Geometry: final body of the model. Coordinates: model frame, mm. Face numbers are marked on the shaded views. A direction names the side the tool comes from. Give positions to 0.01 mm unless a question says otherwise; leave off trailing zeros. Write each loop counter-clockwise with the first axis right and the second up, starting at its lowest first coordinate (ties: lowest second). Pieces come first, ordered by that corner, then holes. Notation, with made-up numbers: (78.5, 59) -> (108.5, 59) arc R11 cw to (108.5, 78) -> close; hole circle Ø7 at (-40, -22). An arc over 180 degrees is marked (long way). Answer as a JSON object with one key per item and string values.
from build123d import *

# Parameters (mm, degrees)
SKETCH1_W           = 154
SKETCH1_H           = 116
BOSS_EXTRUDE1_DEPTH = 70
SKETCH2_W           = 150
SKETCH2_H           = 102
CUT_EXTRUDE1_DEPTH  = 68
SKETCH3_W           = 140
SKETCH3_H           = 5
CUT_EXTRUDE2_DEPTH  = 68
SKETCH5_W           = 70
SKETCH5_H           = 56
CUT_EXTRUDE4_DEPTH  = 5
SKETCH17_W          = 9
SKETCH17_H          = 11
CUT_EXTRUDE12_DEPTH = 178.110135227
FILLET1_R           = 2
FILLET3_R           = 5
FILLET4_R           = 3
FILLET5_R           = 3
FILLET6_R           = 3
FILLET7_R           = 3
FILLET9_R           = 3
FILLET11_R          = 2
FILLET12_R          = 3
FILLET13_R          = 2
SKETCH18_W          = 154
SKETCH18_H          = 116
CUT_EXTRUDE13_DEPTH = 4
SKETCH19_R          = 5
CUT_EXTRUDE14_DEPTH = 4
SKETCH20_R          = 3.5
BOSS_EXTRUDE3_DEPTH = 19.5
SKETCH22_R          = 3.5
BOSS_EXTRUDE4_DEPTH = 18
SKETCH24_R          = 3.25
CUT_EXTRUDE17_DEPTH = 149.882504009
SKETCH25_R          = 3.25
CUT_EXTRUDE18_DEPTH = 176.567650779
SKETCH6_R           = 1.5
CUT_EXTRUDE19_DEPTH = 60
SKETCH26_R          = 2.1
CUT_EXTRUDE20_DEPTH = 10
SKETCH23_R          = 1.5
CUT_EXTRUDE21_DEPTH = 15
SKETCH27_R          = 2.1
CUT_EXTRUDE22_DEPTH = 10
SKETCH21_R          = 1.5
CUT_EXTRUDE23_DEPTH = 15
SKETCH28_R          = 2.1
CUT_EXTRUDE24_DEPTH = 10


with BuildPart() as part:
    # Sketch1 → Boss-Extrude1 (new body)
    with BuildSketch(Plane(origin=(0, 0, 0), x_dir=(1, 0, 0), z_dir=(0, 1, 0))):
        Rectangle(SKETCH1_W, SKETCH1_H)
    extrude(amount=BOSS_EXTRUDE1_DEPTH)

    # Sketch2 → Cut-Extrude1 (cut)
    with BuildSketch(Plane(origin=(0, 70, 0), x_dir=(1, 0, 0), z_dir=(0, 1, 0))):
        Rectangle(SKETCH2_W, SKETCH2_H)
    extrude(amount=-CUT_EXTRUDE1_DEPTH, mode=Mode.SUBTRACT)

    # Sketch3 → Cut-Extrude2 (cut)
    with BuildSketch(Plane(origin=(0, 70, 0), x_dir=(1, 0, 0), z_dir=(0, 1, 0))):
        with Locations((0, 53.5)):
            Rectangle(SKETCH3_W, SKETCH3_H)
    extrude(amount=-CUT_EXTRUDE2_DEPTH, mode=Mode.SUBTRACT)

    # Sketch5 → Cut-Extrude4 (cut)
    with BuildSketch(Plane.XY.offset(58)):
        with Locations((35, 35)):
            Rectangle(SKETCH5_W, SKETCH5_H)
        with Locations((-35, 35)):
            Rectangle(SKETCH5_W, SKETCH5_H)
    extrude(amount=-CUT_EXTRUDE4_DEPTH, mode=Mode.SUBTRACT)

    # Sketch17 → Cut-Extrude12 (cut, through all)
    with BuildSketch(Plane.ZY.offset(-75)):
        with Locations((45.3, 27.5)):
            Rectangle(SKETCH17_W, SKETCH17_H)
    extrude(amount=-CUT_EXTRUDE12_DEPTH, mode=Mode.SUBTRACT)

    # Fillet1
    fillet1_edges = [part.edges().sort_by_distance(p)[0] for p in [
        (77, 27.5, 49.8),
        (77, 22, 45.3),
        (77, 27.5, 40.8),
        (77, 33, 45.3),
    ]]
    fillet(fillet1_edges, radius=FILLET1_R - 0.0001)  # a hair under: the kernel refuses the full size

    # Fillet3
    fillet3_edges = [part.edges().sort_by_distance(p)[0] for p in [
        (0, 7, 53),
        (70, 35, 53),
        (-70, 35, 53),
        (0, 63, 53),
    ]]
    fillet(fillet3_edges, radius=FILLET3_R - 0.0001)  # a hair under: the kernel refuses the full size

    # Fillet4
    fillet4_edges = [part.edges().sort_by_distance(p)[0] for p in [
        (77, 35, 58),
    ]]
    fillet(fillet4_edges, radius=FILLET4_R)

    # Fillet5
    fillet5_edges = [part.edges().sort_by_distance(p)[0] for p in [
        (-77, 35, 58),
    ]]
    fillet(fillet5_edges, radius=FILLET5_R)

    # Fillet6
    fillet6_edges = [part.edges().sort_by_distance(p)[0] for p in [
        (-77, 35, -58),
    ]]
    fillet(fillet6_edges, radius=FILLET6_R)

    # Fillet7
    fillet7_edges = [part.edges().sort_by_distance(p)[0] for p in [
        (77, 35, -58),
    ]]
    fillet(fillet7_edges, radius=FILLET7_R)

    # Fillet9
    fillet9_edges = [part.edges().sort_by_distance(p)[0] for p in [
        (-70, 36, -51),
    ]]
    fillet(fillet9_edges, radius=FILLET9_R)

    # Fillet11
    fillet11_edges = [part.edges().sort_by_distance(p)[0] for p in [
        (-70, 36, -56),
    ]]
    fillet(fillet11_edges, radius=FILLET11_R - 0.0001)  # a hair under: the kernel refuses the full size

    # Fillet12
    fillet12_edges = [part.edges().sort_by_distance(p)[0] for p in [
        (70, 36, -51),
    ]]
    fillet(fillet12_edges, radius=FILLET12_R)

    # Fillet13
    fillet13_edges = [part.edges().sort_by_distance(p)[0] for p in [
        (70, 36, -56),
    ]]
    fillet(fillet13_edges, radius=FILLET13_R - 0.0001)  # a hair under: the kernel refuses the full size

    # Sketch18 → Cut-Extrude13 (cut)
    with BuildSketch(Plane(origin=(0, 70, 0), x_dir=(1, 0, 0), z_dir=(0, 1, 0))):
        Rectangle(SKETCH18_W, SKETCH18_H)
    extrude(amount=-CUT_EXTRUDE13_DEPTH, mode=Mode.SUBTRACT)

    # Sketch19 → Cut-Extrude14 (cut)
    with BuildSketch(Plane(origin=(0, 0, 51), x_dir=(-1, 0, 0), z_dir=(0, 0, -1))):
        with Locations((-13.5, 34)):
            Circle(SKETCH19_R)
        with Locations((4.25, 34)):
            Circle(SKETCH19_R)
        with Locations((22, 34)):
            Circle(SKETCH19_R)
    extrude(amount=-CUT_EXTRUDE14_DEPTH, mode=Mode.SUBTRACT)

    # Sketch20 → Boss-Extrude3 (add)
    with BuildSketch(Plane(origin=(0, 2, 0), x_dir=(1, 0, 0), z_dir=(0, 1, 0))):
        with Locations(Location((-60, -36, 0), (0, 0, 270))):
            Circle(SKETCH20_R)
        with Locations(Location((8, -40, 0), (0, 0, 270))):
            Circle(SKETCH20_R)
        with Locations(Location((-59, 33, 0), (0, 0, 270))):
            Circle(SKETCH20_R)
        with Locations(Location((20, 34, 0), (0, 0, 270))):
            Circle(SKETCH20_R)
    extrude(amount=BOSS_EXTRUDE3_DEPTH)

    # Sketch22 → Boss-Extrude4 (add)
    with BuildSketch(Plane(origin=(0, 2, 0), x_dir=(1, 0, 0), z_dir=(0, 1, 0))):
        with Locations(Location((50, 29, 0), (0, 0, 270))):
            Circle(SKETCH22_R)
        with Locations(Location((35, 3, 0), (0, 0, 270))):
            Circle(SKETCH22_R)
        with Locations(Location((67, 3, 0), (0, 0, 270))):
            Circle(SKETCH22_R)
        with Locations(Location((54, -44, 0), (0, 0, 270))):
            Circle(SKETCH22_R)
    extrude(amount=BOSS_EXTRUDE4_DEPTH)

    # Sketch24 → Cut-Extrude17 (cut, through all)
    with BuildSketch(Plane(origin=(0, 0, 51), x_dir=(-1, 0, 0), z_dir=(0, 0, -1))):
        with Locations((-35, 24.5)):
            Circle(SKETCH24_R)
    extrude(amount=-CUT_EXTRUDE17_DEPTH, mode=Mode.SUBTRACT)

    # Sketch25 → Cut-Extrude18 (cut, through all)
    with BuildSketch(Plane(origin=(-75, 0, 0), x_dir=(0, 0, -1), z_dir=(1, 0, 0))):
        with Locations((-44, 24.5)):
            Circle(SKETCH25_R)
        with Locations((41.2, 24.5)):
            Circle(SKETCH25_R)
    extrude(amount=-CUT_EXTRUDE18_DEPTH, mode=Mode.SUBTRACT)

    # Sketch6 → Cut-Extrude19 (cut)
    with BuildSketch(Plane(origin=(0, 70, 0), x_dir=(1, 0, 0), z_dir=(0, 1, 0))):
        with Locations(Location((73.5, 54.5, 0), (0, 0, 270))):
            Circle(SKETCH6_R)
        with Locations(Location((-73.5, 54.5, 0), (0, 0, 270))):
            Circle(SKETCH6_R)
        with Locations(Location((73.5, -54.5, 0), (0, 0, 270))):
            Circle(SKETCH6_R)
        with Locations(Location((-73.5, -54.5, 0), (0, 0, 270))):
            Circle(SKETCH6_R)
    extrude(amount=-CUT_EXTRUDE19_DEPTH, mode=Mode.SUBTRACT)

    # Sketch26 → Cut-Extrude20 (cut)
    with BuildSketch(Plane(origin=(0, 66, 0), x_dir=(1, 0, 0), z_dir=(0, 1, 0))):
        with Locations(Location((73.5, -54.5, 0), (0, 0, 270))):
            Circle(SKETCH26_R)
        with Locations(Location((73.5, 54.5, 0), (0, 0, 270))):
            Circle(SKETCH26_R)
        with Locations(Location((-73.5, 54.5, 0), (0, 0, 270))):
            Circle(SKETCH26_R)
        with Locations(Location((-73.5, -54.5, 0), (0, 0, 270))):
            Circle(SKETCH26_R)
    extrude(amount=-CUT_EXTRUDE20_DEPTH, mode=Mode.SUBTRACT)

    # Sketch23 → Cut-Extrude21 (cut)
    with BuildSketch(Plane(origin=(0, 20, 0), x_dir=(1, 0, 0), z_dir=(0, 1, 0))):
        with Locations(Location((35, 3, 0), (0, 0, 270))):
            Circle(SKETCH23_R)
        with Locations(Location((50, 29, 0), (0, 0, 270))):
            Circle(SKETCH23_R)
        with Locations(Location((67, 3, 0), (0, 0, 270))):
            Circle(SKETCH23_R)
        with Locations(Location((54, -44, 0), (0, 0, 270))):
            Circle(SKETCH23_R)
    extrude(amount=-CUT_EXTRUDE21_DEPTH, mode=Mode.SUBTRACT)

    # Sketch27 → Cut-Extrude22 (cut)
    with BuildSketch(Plane(origin=(0, 20, 0), x_dir=(1, 0, 0), z_dir=(0, 1, 0))):
        with Locations(Location((54, -44, 0), (0, 0, 270))):
            Circle(SKETCH27_R)
        with Locations(Location((35, 3, 0), (0, 0, 270))):
            Circle(SKETCH27_R)
        with Locations(Location((50, 29, 0), (0, 0, 270))):
            Circle(SKETCH27_R)
        with Locations(Location((67, 3, 0), (0, 0, 270))):
            Circle(SKETCH27_R)
    extrude(amount=-CUT_EXTRUDE22_DEPTH, mode=Mode.SUBTRACT)

    # Sketch21 → Cut-Extrude23 (cut)
    with BuildSketch(Plane(origin=(0, 21.5, 0), x_dir=(1, 0, 0), z_dir=(0, 1, 0))):
        with Locations(Location((-59, 33, 0), (0, 0, 270))):
            Circle(SKETCH21_R)
        with Locations(Location((20, 34, 0), (0, 0, 270))):
            Circle(SKETCH21_R)
        with Locations(Location((8, -40, 0), (0, 0, 270))):
            Circle(SKETCH21_R)
        with Locations(Location((-60, -36, 0), (0, 0, 270))):
            Circle(SKETCH21_R)
    extrude(amount=-CUT_EXTRUDE23_DEPTH, mode=Mode.SUBTRACT)

    # Sketch28 → Cut-Extrude24 (cut)
    with BuildSketch(Plane(origin=(0, 21.5, 0), x_dir=(1, 0, 0), z_dir=(0, 1, 0))):
        with Locations(Location((-59, 33, 0), (0, 0, 270))):
            Circle(SKETCH28_R)
        with Locations(Location((-60, -36, 0), (0, 0, 270))):
            Circle(SKETCH28_R)
        with Locations(Location((8, -40, 0), (0, 0, 270))):
            Circle(SKETCH28_R)
        with Locations(Location((20, 34, 0), (0, 0, 270))):
            Circle(SKETCH28_R)
    extrude(amount=-CUT_EXTRUDE24_DEPTH, mode=Mode.SUBTRACT)


solid = part.part
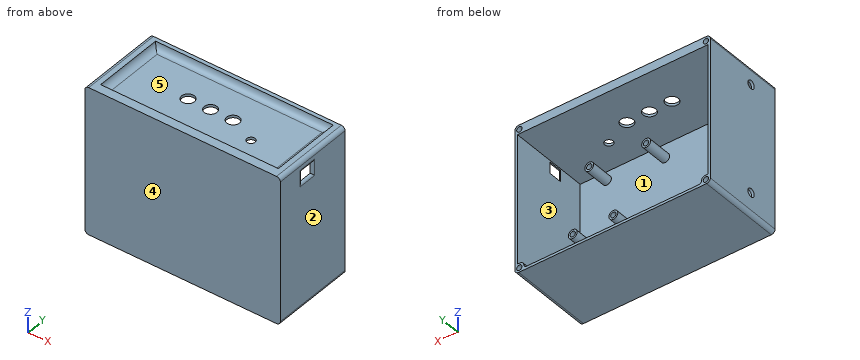
Q1. Mould query, pull axis Z, two halves, no side actions, for the marked faces 3, 4 and 5. Classes: pulls with the +Z half, pulls with the -Z half, needs draft (parallel to the pull), parting line crosses it, or undercut.
Values:
{"face 3": "undercut", "face 4": "needs draft", "face 5": "pulls with the +Z half"}
Q2. Set-up query: the marked faces 1 and 2. Return all of +Z, -Z, +X, -X, +Y, -Y with unobstructed straight access to the full face (end or side cutting, diameter ignored); none if empty.
Values:
{"face 1": "+Y", "face 2": "+Z, -Z, +X, +Y, -Y"}
Q3. First-contact query: P1, Ø5.5, axis at x = -57.5, z = -32, coming from the +Y side; P2, Ø6, axis at x = 24, z = 40, coming from the -Y side; P3, Ø16, axis at x = -22, y = 34, coming from the +Z side; P4, Ø6, axis at y = 24.5, z = 44, coming from the +X side. Flat tips, straight axial feed; report the tip coordinate or a pass-through.
Values:
{"P1": "y = 21.5", "P2": "y = 0", "P3": "z = 53", "P4": "x = 76.32"}
Q4. Material intervals for L1, parallel to Z at x = -18.5, y = 39; L2, parallel to X at y = 35, z = 0.5; L3, parallel to X at y = 15, z = 40, sorted ascending. Write a range as from..to.
Values:
{"L1": "-58..-56, 51..53", "L2": "-77..-75, 75..77", "L3": "-77..-75, 4.5..5.9, 10.1..11.5, 75..77"}
Q5. Cut plane C-C (z = 30). Return the cut outline in (x, y).
Values:
{"outline": "(-77, 0) -> (77, 0) -> (77, 66) -> (75, 66) -> (75, 2) -> (-75, 2) -> (-75, 66) -> (-77, 66) -> close"}
Q6. Cut plane B-B (y = 24.5). State how many separate pieces and enclosed holes the cut face has, and give its area (3 significant figures).
Values:
{"separate pieces": "4", "enclosed holes": "4", "area": "1,080 mm²"}
